Geometry: final body of the model. Coordinates: model frame, mm. A direction names the side the tool comes from. Give positions to 0.01 mm unless a question says otherwise; leave off trailing zeros. Write each loop counter-clockwise with the first axis right and the second up, starting at its lowest first coordinate (ties: lowest second). Pieces come first, ordered by that corner, then holes. Notation, with made-up numbers: M -12.5,32 L 10.5,32 A24 cw 10.5,44 Z; hole C 38.5,83.25 d10. An arc over 180 degrees is marked long. One line per question, with ' | ' between items.
from build123d import *

# Parameters (mm, degrees)
F0_W     = 38.1
F0_H     = 19.05
F1_DEPTH = 3.175
F2_R     = 2.81996
F3_DEPTH = 3.176
F5_DEPTH = 1.27
F6_DEPTH = 2.032


with BuildPart() as f1:
    # F0 (on Top) → F1 (new body)
    with BuildSketch(Plane.XY):
        with Locations((-19.05, 9.525)):
            Rectangle(F0_W, F0_H)
    extrude(amount=F1_DEPTH)

    # F2 (on face) → F3 (cut, through all)
    with BuildSketch(Plane.XY.offset(3.175)):
        with BuildLine():
            ThreePointArc((-38.1, 9.525), (-35.381374, 16.053134), (-28.9762, 19.05))
            Line((-28.9762, 19.05), (-38.1, 19.05))
            Line((-38.1, 19.05), (-38.1, 9.525))
        make_face()
        with BuildLine():
            ThreePointArc((-28.9762, 0), (-35.381374, 2.996866), (-38.1, 9.525))
            Line((-38.1, 9.525), (-38.1, 0))
            Line((-38.1, 0), (-28.9762, 0))
        make_face()
        with Locations((-31.952918, 9.525)):
            Circle(F2_R)
    extrude(amount=-F3_DEPTH, mode=Mode.SUBTRACT)

    # F4 (on face) → F5 (join)
    with BuildSketch(Plane.XY.offset(3.175)):
        with BuildLine():
            ThreePointArc((-15.194452, 18.448619), (-19.817669, 16.003864), (-20.874732, 10.881991))
            Line((-20.874732, 10.881991), (-20.671532, 10.881991))
            Line((-20.671532, 10.881991), (-20.320076, 10.963324))
            Line((-20.320076, 10.963324), (-19.771464, 11.066189))
            Line((-19.771464, 11.066189), (-19.291429, 11.160482))
            Line((-19.291429, 11.160482), (-18.911961, 11.260434))
            Line((-18.911961, 11.260434), (-18.586872, 11.327949))
            Line((-18.586872, 11.327949), (-18.261783, 11.327949))
            Line((-18.261783, 11.327949), (-17.762255, 11.327949))
            Line((-17.762255, 11.327949), (-17.223081, 11.327949))
            Line((-17.223081, 11.327949), (-16.794914, 11.327949))
            Line((-16.794914, 11.327949), (-16.431164, 11.260434))
            Line((-16.431164, 11.260434), (-16.233785, 11.225344))
            Line((-16.233785, 11.225344), (-15.955806, 11.155849))
            Line((-15.955806, 11.155849), (-15.720593, 11.086354))
            Line((-15.720593, 11.086354), (-15.498744, 10.979439))
            Line((-15.498744, 10.979439), (-15.327681, 10.872524))
            Line((-15.327681, 10.872524), (-15.15326, 10.739213))
            Line((-15.15326, 10.739213), (-15.022739, 10.64253))
            Line((-15.022739, 10.64253), (-14.872882, 10.758549))
            Line((-14.872882, 10.758549), (-14.649567, 10.92315))
            Line((-14.649567, 10.92315), (-14.321024, 11.11269))
            Line((-14.321024, 11.11269), (-14.07626, 11.221474))
            Line((-14.07626, 11.221474), (-13.782543, 11.308501))
            Line((-13.782543, 11.308501), (-13.477948, 11.352015))
            Line((-13.477948, 11.352015), (-13.238624, 11.352015))
            Line((-13.238624, 11.352015), (-12.885077, 11.352015))
            Line((-12.885077, 11.352015), (-12.553286, 11.352015))
            Line((-12.553286, 11.352015), (-12.145346, 11.352015))
            Line((-12.145346, 11.352015), (-11.748285, 11.352015))
            Line((-11.748285, 11.352015), (-11.356664, 11.352015))
            Line((-11.356664, 11.352015), (-10.986798, 11.308501))
            Line((-10.986798, 11.308501), (-10.790988, 11.264987))
            Line((-10.790988, 11.264987), (-10.470076, 11.216035))
            Line((-10.470076, 11.216035), (-10.132845, 11.139886))
            Line((-10.132845, 11.139886), (-9.730345, 11.031102))
            Line((-9.730345, 11.031102), (-9.210265, 10.879805))
            ThreePointArc((-9.210265, 10.879805), (-10.357813, 16.122579), (-15.194452, 18.448619))
        make_face()
    extrude(amount=F5_DEPTH)

    # F4 (on face) → F6 (join)
    with BuildSketch(Plane.XY.offset(3.175)):
        with BuildLine():
            Line((-23.068097, 10.490683), (-23.225745, 10.490683))
            Line((-23.225745, 10.490683), (-23.225745, 1.513947))
            Line((-23.225745, 1.513947), (-16.128955, 1.513947))
            ThreePointArc((-16.128955, 1.513947), (-15.046753, 1.367138), (-13.964551, 1.513947))
            Line((-13.964551, 1.513947), (-6.886078, 1.513947))
            Line((-6.886078, 1.513947), (-6.886078, 10.435192))
            Line((-6.886078, 10.435192), (-7.009125, 10.435192))
            Line((-7.009125, 10.435192), (-7.190363, 10.616429))
            Line((-7.190363, 10.616429), (-7.648225, 10.616429))
            Line((-7.648225, 10.616429), (-8.058394, 10.616429))
            Line((-8.058394, 10.616429), (-8.506718, 10.69274))
            Line((-8.506718, 10.69274), (-8.850115, 10.778589))
            Line((-8.850115, 10.778589), (-9.210265, 10.879805))
            Line((-9.210265, 10.879805), (-9.730345, 11.031102))
            Line((-9.730345, 11.031102), (-10.132845, 11.139886))
            Line((-10.132845, 11.139886), (-10.470076, 11.216035))
            Line((-10.470076, 11.216035), (-10.790988, 11.264987))
            Line((-10.790988, 11.264987), (-10.986798, 11.308501))
            Line((-10.986798, 11.308501), (-11.356664, 11.352015))
            Line((-11.356664, 11.352015), (-11.748285, 11.352015))
            Line((-11.748285, 11.352015), (-12.145346, 11.352015))
            Line((-12.145346, 11.352015), (-12.553286, 11.352015))
            Line((-12.553286, 11.352015), (-12.885077, 11.352015))
            Line((-12.885077, 11.352015), (-13.238624, 11.352015))
            Line((-13.238624, 11.352015), (-13.477948, 11.352015))
            Line((-13.477948, 11.352015), (-13.782543, 11.308501))
            Line((-13.782543, 11.308501), (-14.07626, 11.221474))
            Line((-14.07626, 11.221474), (-14.321024, 11.11269))
            Line((-14.321024, 11.11269), (-14.649567, 10.92315))
            Line((-14.649567, 10.92315), (-14.872882, 10.758549))
            Line((-14.872882, 10.758549), (-15.022739, 10.64253))
            Line((-15.022739, 10.64253), (-15.15326, 10.739213))
            Line((-15.15326, 10.739213), (-15.327681, 10.872524))
            Line((-15.327681, 10.872524), (-15.498744, 10.979439))
            Line((-15.498744, 10.979439), (-15.720593, 11.086354))
            Line((-15.720593, 11.086354), (-15.955806, 11.155849))
            Line((-15.955806, 11.155849), (-16.233785, 11.225344))
            Line((-16.233785, 11.225344), (-16.431164, 11.260434))
            Line((-16.431164, 11.260434), (-16.794914, 11.327949))
            Line((-16.794914, 11.327949), (-17.223081, 11.327949))
            Line((-17.223081, 11.327949), (-17.762255, 11.327949))
            Line((-17.762255, 11.327949), (-18.261783, 11.327949))
            Line((-18.261783, 11.327949), (-18.586872, 11.327949))
            Line((-18.586872, 11.327949), (-18.911961, 11.260434))
            Line((-18.911961, 11.260434), (-19.291429, 11.160482))
            Line((-19.291429, 11.160482), (-19.771464, 11.066189))
            Line((-19.771464, 11.066189), (-20.320076, 10.963324))
            Line((-20.320076, 10.963324), (-20.671532, 10.881991))
            Line((-20.671532, 10.881991), (-20.874732, 10.881991))
            Line((-20.874732, 10.881991), (-21.348417, 10.795149))
            Line((-21.348417, 10.795149), (-21.751048, 10.700412))
            Line((-21.751048, 10.700412), (-22.276284, 10.614889))
            Line((-22.276284, 10.614889), (-22.866262, 10.614889))
            Line((-22.866262, 10.614889), (-23.068097, 10.490683))
        make_face()
    extrude(amount=F6_DEPTH)


solid = f1.part
(1) First-contact query: P1, Ø0.6, axis at y = 6, z = 4, coming from the +X side; P2, Ø1, axis at x = -20, z = 4, coming from the -Y side; P3, Ø0.8, axis at x = -12, z = 4.5, coming from the +Y side; P4, Ø4.5, axis at x = -31.95, y = 9.52, coming from the +Z side. Flat tips, straight axial feed; report the tip coordinate or a pass-through.
Working result:
P1: stops at x = -6.89 | P2: stops at y = 1.51 | P3: stops at y = 17.79 | P4: passes through
(2) Draft query along Y for faces 1 (the face through (-34.19, 7.81, 1.61)), 2 (the face through (0, 9, 2)), 3 (the face through (-35.45, 15.98, 1.61)). Return one class per face: released by +Y, released by -Y, zero draft, split by the parting line, or undercut.
Working result:
face 1: undercut | face 2: zero draft | face 3: released by +Y
(3) Cut plane A-A, the plane y = 8. Return loops of the section in (x, z) (3 decimals), then the cut area to 3 significant figures.
Working result:
outline: M -37.941,0 L -34.325,0 L -34.325,3.175 L -37.941,3.175 Z; M -29.581,0 L 0,0 L 0,3.175 L -6.886,3.175 L -6.886,5.207 L -23.226,5.207 L -23.226,3.175 L -29.581,3.175 Z | area: 139 mm^2
(4) Material intervals for L1, parallel to X at y = 10, z = 3.85; L2, parallel to Z at x = -34, y = 15 (3 decimals); L3, parallel to X at y = 10, z = 3.1, sorted ascending. Write a range as [from, to].
Working result:
L1: x = [-23.23, -6.89] | L2: z = [0, 3.175] | L3: x = [-38.08, -34.73], [-29.17, 0]
(5) Set-up query: faces 4 (the face through (-6.886, 6, 4)), 5 (the face through (-7.6, 10.616, 4.2)), 6 (the face through (-15.062, 1.367, 4.177)). Return all of +Z, -Z, +X, -X, +Y, -Y with unobstructed straight access to the full face (end or side cutting, diameter ignored); none if empty.
Working result:
face 4: +Z, +X, +Y, -Y | face 5: +Z, +X, +Y | face 6: +Z, -Y
(6) Cut plane C-C, the plane z = 4. Return loops of the section in (x, y).
Working result:
outline: M -23.23,1.51 L -16.13,1.51 A4.06 ccw -13.96,1.51 L -6.89,1.51 L -6.89,10.44 L -7.01,10.44 L -7.19,10.62 L -8.06,10.62 L -8.51,10.69 L -8.85,10.78 L -9.21,10.88 A6.12 ccw -15.19,18.45 A6.13 ccw -20.87,10.88 L -21.35,10.8 L -21.75,10.7 L -22.28,10.61 L -22.87,10.61 L -23.07,10.49 L -23.23,10.49 Z
(7) Cut plane D-D, the plane y = 4. Return loops of the section in (x, z) (3 decimals).
Working result:
outline: M -36.221,0 L 0,0 L 0,3.175 L -6.886,3.175 L -6.886,5.207 L -23.226,5.207 L -23.226,3.175 L -36.221,3.175 Z
(8) Cut plane B-B, the plane x = -30. Return loops of the section in (y, z) (1 decimal).
Working result:
outline: M 0.1,0 L 7.5,0 L 7.5,3.2 L 0.1,3.2 Z; M 11.6,0 L 18.9,0 L 18.9,3.2 L 11.6,3.2 Z
